from build123d import *
from build123d.topology import SkipClean

# Parameters (mm, degrees)
SKETCH_2_R          = 2.1
SKETCH_2_R_2        = 4
EXTRUDE_2_DEPTH     = 4
SKETCH_2_4_R        = 2.1
SKETCH_2_4_R_2      = 4
CUT_EXTRUDE_1_DEPTH = 15


with BuildPart() as part:
    # 草图2 → 凸台-拉伸2 (new body)
    with BuildSketch(Plane.XY):
        Polygon((-51.411814067, -23.645961981), (183.493005706, -23.645961981), (183.493005706, 28.798986499), (106.485233254, 28.798986499), (106.485233254, 83.235515302), (73, 83.235515302), (73, 165.222238559), (8.133015227, 260.154233909), (-51.411814067, 260.154233909), align=None)
        with Locations((6.416988046, 8.689671313)):
            Circle(SKETCH_2_R, mode=Mode.SUBTRACT)
        with Locations((-5.491997211, 19.849072718)):
            Circle(SKETCH_2_R, mode=Mode.SUBTRACT)
        with Locations((-14.493242982, 33.462806377)):
            Circle(SKETCH_2_R, mode=Mode.SUBTRACT)
        with BuildLine():
            Line((24.119237886, 0), (22.019237886, 0))
            ThreePointArc((22.019237886, 0), (22.997160887, -0.38239852), (23.980709842, -0.750085173))
            ThreePointArc((23.980709842, -0.750085173), (19.954160272, 0.381384906), (24.119237886, 0))
        make_face(mode=Mode.SUBTRACT)
        with BuildLine():
            ThreePointArc((52, -5), (47.94285131, -8.999591733), (44.001632986, -4.885714286))
            ThreePointArc((44.001632986, -4.885714286), (46, -4.971422738), (48, -5))
            Line((48, -5), (52, -5))
        make_face(mode=Mode.SUBTRACT)
        with Locations((-22, 65)):
            Circle(SKETCH_2_R, mode=Mode.SUBTRACT)
        with Locations((-20.097455932, 48.790851483)):
            Circle(SKETCH_2_R, mode=Mode.SUBTRACT)
        with Locations((48, 65)):
            Circle(SKETCH_2_R_2, mode=Mode.SUBTRACT)
        with BuildLine():
            ThreePointArc((77, -5), (73, -9), (69, -5))
            Line((69, -5), (77, -5))
        make_face(mode=Mode.SUBTRACT)
        with BuildLine():
            ThreePointArc((102, -5), (98, -9), (94, -5))
            Line((94, -5), (102, -5))
        make_face(mode=Mode.SUBTRACT)
        with BuildLine():
            ThreePointArc((127, -5), (123, -9), (119, -5))
            Line((119, -5), (127, -5))
        make_face(mode=Mode.SUBTRACT)
        with Locations((148, -5)):
            Circle(SKETCH_2_R_2, mode=Mode.SUBTRACT)
        with Locations((90, 65)):
            Circle(SKETCH_2_R_2, mode=Mode.SUBTRACT)
        with Locations((48, 135)):
            Circle(SKETCH_2_R_2, mode=Mode.SUBTRACT)
        with BuildLine():
            ThreePointArc((-2.118495143, 207.333508449), (-7.684495307, 208.343281781), (-6.674721974, 213.909281945))
            ThreePointArc((-6.674721974, 213.909281945), (-1.108721811, 212.899508613), (-2.118495143, 207.333508449))
        make_face(mode=Mode.SUBTRACT)
        with Locations((8.133015227, 192.538018085)):
            Circle(SKETCH_2_R_2, mode=Mode.SUBTRACT)
    extrude(amount=EXTRUDE_2_DEPTH)

    # 草图2<4> → 切除-拉伸1 (cut, symmetric)
    with SkipClean():  # the faces are left unmerged after this step: merging them gives an invalid solid
        with BuildSketch(Plane.XY):
            with Locations((6.416988046, 8.689671313)):
                Circle(SKETCH_2_4_R)
            with Locations((-22, 65)):
                Circle(SKETCH_2_4_R)
            with Locations((-14.493242982, 33.462806377)):
                Circle(SKETCH_2_4_R)
            with Locations((22.019237886, 0)):
                Circle(SKETCH_2_4_R)
            with Locations((-20.097455932, 48.790851483)):
                Circle(SKETCH_2_4_R)
            with Locations((-5.491997211, 19.849072718)):
                Circle(SKETCH_2_4_R)
            with Locations((48, -5)):
                Circle(SKETCH_2_4_R_2)
            with Locations((148, -5)):
                Circle(SKETCH_2_4_R_2)
            with Locations((98, -5)):
                Circle(SKETCH_2_4_R_2)
            with Locations((73, -5)):
                Circle(SKETCH_2_4_R_2)
            with Locations((123, -5)):
                Circle(SKETCH_2_4_R_2)
        extrude(amount=CUT_EXTRUDE_1_DEPTH, both=True, mode=Mode.SUBTRACT)


solid = part.part
Read the model definition and answer for the solid it produces. Units are mm, in the model's axes. Give positions to 0.01 mm unless a question says otherwise; leave off trailing zeros. Write each loop counter-clockwise with the first axis right and the second up, starting at its lowest first coordinate (ties: lowest second). Pieces come first, ordered by that corner, then holes. Notation, with made-up numbers: (30, -24) - (88, -24) arc R22 cw to (88, 10) - close; hole circle Ø7 at (-28.5, 83.25). An arc over 180 degrees is marked (long way). Use CSV: the item, a comma, the result in double quotes. Start each with the question number.
Item 1: The part is cut by section A-A, the plane y = 135. Give the vertices of the cut face in (x, z).
Item 2: The part is cut by section B-B, the plane x = 148. Give the vertices of the cut face in (y, z), and give its area (3 significant figures).
Item 3: The mould has two halves that part along X. Classify faces 1 (the cylindrical face through (47.133, 61.095, 1.972)), 2 (the flat face through (41.021, 212.024, 1.972)), 3 (the cylindrical face through (7.266, 188.633, 1.972)), 4 (the flat face through (38, 89, 0)): pulls with the +X half, pulls with the -X half, needs draft (parallel to the pull), parting line crosses it, or undercut.
Item 4: The part is cut by section D-D, the plane x = 48. Give the vertices of the cut face in (y, z).
Item 5: Flat-ended cylindrical pins translate along their axes: P1, Ø3.5, axis at x = -14.49, y = 33.46, coming from the -Z side; P2, Ø5.5, axis at x = -5.49, y = 19.85, coming from the -Z side; P3, Ø1.2, axis at y = 128.5, z = 2, coming from the +X side; P4, Ø1.5, axis at y = 50.5, z = 1.5, coming from the +X side. Find the tip coordinate at first contact, or state that the pin passes through.
Item 6: Consider line 1 (Y direction, x = -6, z = 2.05); line 2 (Y direction, x = 45, z = 0.8); line 3 (X direction, y = 110, z = 1.65). Determine where each line is inside the solid, lowest interval first.
Taken from the geometry:
1,outline,"(-51.41, 0) - (44, 0) - (44, 4) - (-51.41, 4) - close; (52, 0) - (73, 0) - (73, 4) - (52, 4) - close"
2,outline,"(-23.65, 0) - (-9, 0) - (-9, 4) - (-23.65, 4) - close; (-1, 0) - (28.8, 0) - (28.8, 4) - (-1, 4) - close"
2,area,"178 mm2"
3,face 1,"undercut"
3,face 2,"pulls with the +X half"
3,face 3,"undercut"
3,face 4,"needs draft"
4,outline,"(-23.65, 0) - (-9, 0) - (-9, 4) - (-23.65, 4) - close; (-1, 0) - (61, 0) - (61, 4) - (-1, 4) - close; (69, 0) - (131, 0) - (131, 4) - (69, 4) - close; (139, 0) - (201.81, 0) - (201.81, 4) - (139, 4) - close"
5,P1,"through"
5,P2,"z = 0"
5,P3,"x = 73"
5,P4,"x = 106.49"
6,line 1,"-23.65 to 17.81, 21.89 to 206.96, 214.29 to 260.15"
6,line 2,"-23.65 to -7.65, -2.35 to 62.35, 67.65 to 132.35, 137.65 to 206.2"
6,line 3,"-51.41 to 73"
